```python
from build123d import *

# Parameters (mm, degrees)
SKETCH_1_R          = 16
EXTRUDE_1_DEPTH     = 24
SKETCH_2_R          = 8.5
CUT_EXTRUDE_1_DEPTH = 14
SKETCH_3_R          = 3
CUT_EXTRUDE_2_DEPTH = 20
SKETCH_4_R          = 9.5
CUT_EXTRUDE_4_DEPTH = 14
CHAMFER_1_SIZE      = 0.5
CHAMFER_1_SIZE2     = 0.866025404
CHAMFER_2_SIZE      = 1.5
CHAMFER_2_SIZE2     = 0.401923789
M3X0_51_D           = 2.5
M3X0_51_DEPTH       = 5.5
M3X0_51_TIP         = 0.751075774
CHAMFER_3_SIZE      = 0.5


with BuildPart() as part:
    # Эскиз1 → Бобышка-Вытянуть1 (new body)
    with BuildSketch(Plane(origin=(0, 0, 0), x_dir=(1, 0, 0), z_dir=(0, 1, 0))):
        with Locations(Location((0, 0, 0), (0, 0, 270))):
            Circle(SKETCH_1_R)
    extrude(amount=EXTRUDE_1_DEPTH)

    # Эскиз2 → Вырез-Вытянуть1 (cut)
    with BuildSketch(Plane(origin=(0, 24, 0), x_dir=(1, 0, 0), z_dir=(0, 1, 0))):
        with Locations(Location((-5, 0, 0), (0, 0, 270))):
            Circle(SKETCH_2_R)
    extrude(amount=-CUT_EXTRUDE_1_DEPTH, mode=Mode.SUBTRACT)

    # Эскиз3 → Вырез-Вытянуть2 (cut)
    with BuildSketch(Plane(origin=(0, 24, 0), x_dir=(1, 0, 0), z_dir=(0, 1, 0))):
        with Locations(Location((9.6, 0, 0), (0, 0, 270))):
            Circle(SKETCH_3_R)
    extrude(amount=-CUT_EXTRUDE_2_DEPTH, mode=Mode.SUBTRACT)

    # Эскиз4 → Вырез-Вытянуть4 (cut)
    with BuildSketch(Plane(origin=(0, 0, 0), x_dir=(1, 0, 0), z_dir=(0, 1, 0))):
        with Locations(Location((-5, 0, 0), (0, 0, 270))):
            Circle(SKETCH_4_R)
    extrude(amount=CUT_EXTRUDE_4_DEPTH, mode=Mode.SUBTRACT)

    # Фаска1
    chamfer_1_edges = [part.edges().sort_by_distance(p)[0] for p in [
        (-5, 0, -9.5),
    ]]
    chamfer_1_side = [part.faces().sort_by_distance(p)[0] for p in [
        (0, 0, -15.54745166),
    ]]
    chamfer(chamfer_1_edges, length=CHAMFER_1_SIZE, length2=CHAMFER_1_SIZE2, reference=chamfer_1_side[0])

    # Фаска2
    chamfer_2_edges = [part.edges().sort_by_distance(p)[0] for p in [
        (0, 0, -16),
    ]]
    chamfer_2_side = [part.faces().sort_by_distance(p)[0] for p in [
        (0, 12, -16),
    ]]
    chamfer(chamfer_2_edges, length=CHAMFER_2_SIZE, length2=CHAMFER_2_SIZE2, reference=chamfer_2_side[0])

    # Отверстие обработанное метчиком M3x0.51
    with Locations(Plane(origin=(0, 24, 0), x_dir=(1, 0, 0), z_dir=(0, 1, 0))):
        with Locations((0, 10), (0, -10)):
            Hole(M3X0_51_D / 2, depth=M3X0_51_DEPTH)
            with Locations((0, 0, -(M3X0_51_DEPTH + M3X0_51_TIP / 2))):  # 118° drill point
                Cone(0, M3X0_51_D / 2, M3X0_51_TIP, mode=Mode.SUBTRACT)

    # Фаска3
    chamfer_3_edges = [part.edges().sort_by_distance(p)[0] for p in [
        (1.25, 24, 10),
        (1.25, 24, -10),
    ]]
    chamfer(chamfer_3_edges, length=CHAMFER_3_SIZE)


solid = part.part
```
CAD build for the part. Positions are in the model's coordinates, mm. A direction names the side the tool comes from. Coordinates: 2 decimals unless noted, no trailing zeros. Loops run counter-clockwise (first coordinate to the right, second up) from the corner with the lowest first, then second, coordinate; pieces in that order, holes last. Notation, with made-up numbers: (27.5, 45) - (37.5, 45) arc R33 ccw to (37.5, 73) - close; hole circle Ø4 at (24.25, 51.5). An arc over 180 degrees is marked (long way). Use CSV: the item, a comma, the result in double quotes. Start each with the question number.
Q1. 3-axis set-ups, long thin cutter, end or side, ignore diameter. For faces 1 (the flat face through (10, 4, 0)), 2 (the flat face through (-13.4, 14, -2.2)), 3 (the flat face through (4, 24, 0)): which of +Z, -Z, +X, -X, +Y, -Y reach the whole face in a straight line?
Q2. Cut at B-B, the plane y = 22.25. List the corners of the cut face in (x, z).
Q3. Cut at A-A, the plane z = 0. List the corners of the cut face in (x, y).
Q4. Two-plate mould, pull along Z, no slides. Class faces 4 (the cylindrical face through (-2.146, 7.341, 9.061)), 5 (the cylindrical face through (-15.62, 12.59, -3.47)), 6 (the flat face through (7, 0, 0)), 7 (the cylindrical face through (12.574, 14.14, -0.391)): +Z half, -Z half, draft (parallel to the pull), parting line (faces both ways), or undercut.
Q5. Drop flat-ended pins along their axis: P1, Ø8, axis at y = 4.5, z = 11, coming from the -X side; P2, Ø3, axis at x = 0, z = 10, coming from the +Y side; P3, Ø1, axis at y = 19, z = 3.5, coming from the -X side. Give the stop position or say it passes through.
Q6. Cut at D-D, the plane y = 2.5. List the corners of the cut face in (x, z).
Q7. Probe probe 1 along X at (y, z) = (7.5, 0); probe 2 along X at (y, z) = (18, 0); probe 3 along Z at (x, y) = (-9.5, 6.5). List the from-to ranges inside material, lowest first. Write a range as from..to.
Q8. Cut at C-C, the plane y = 9.5. List the corners of the cut face in (x, z).
Here are the results:
1,face 1,"+Y"
1,face 2,"-Y"
1,face 3,"+Z, -Z, +X, -X, +Y"
2,outline,"circle Ø32 at (0, 0); hole circle Ø17 at (-5, 0); hole circle Ø2.5 at (0, -10); hole circle Ø2.5 at (0, 10); hole circle Ø6 at (9.6, 0)"
3,outline,"(-16, 1.5) - (-15.6, 0) - (-15, 0) - (-14.5, 0.87) - (-14.5, 14) - (-13.5, 14) - (-13.5, 24) - (-16, 24) - close; (3.5, 14) - (4.5, 14) - (4.5, 0.87) - (5, 0) - (15.6, 0) - (16, 1.5) - (16, 24) - (12.6, 24) - (12.6, 4) - (6.6, 4) - (6.6, 24) - (3.5, 24) - close"
4,face 4,"undercut"
4,face 5,"parting line"
4,face 6,"draft"
4,face 7,"undercut"
5,P1,"x = -14.39"
5,P2,"y = 23.75"
5,P3,"x = -15.72"
6,outline,"circle Ø32 at (0, 0); hole circle Ø19 at (-5, 0)"
7,probe 1,"-16..-14.5, 4.5..6.6, 12.6..16"
7,probe 2,"-16..-13.5, 3.5..6.6, 12.6..16"
7,probe 3,"-12.87..-8.37, 8.37..12.87"
8,outline,"circle Ø32 at (0, 0); hole circle Ø19 at (-5, 0); hole circle Ø6 at (9.6, 0)"
